from build123d import *

# Parameters (mm, degrees)
F1_DEPTH = 50.8
F2_R     = 7.58365402
F3_DEPTH = 38.1
F4_DEPTH = 38.1
F5_R     = 6.3202279554
F6_DEPTH = 76.2
F7_R     = 6.2629522454
F8_DEPTH = 50.8


with BuildPart() as f1:
    # F0 (on Top) → F1 (new body)
    with BuildSketch(Plane.XY):
        Polygon((-23.0499133468, 13.3078736756), (-23.0499133468, -13.3078736756), (0, -26.6157473511), (23.0499133468, -13.3078736756), (23.0499133468, 13.3078736756), (0, 26.6157473511), align=None)
        Polygon((0, -19.5391465708), (-16.9213972986, -9.7695732854), (-16.9213972986, 9.7695732854), (0, 19.5391465708), (16.9213972986, 9.7695732854), (16.9213972986, -9.7695732854), align=None, mode=Mode.SUBTRACT)
    extrude(amount=F1_DEPTH)

    # F2 (on Right) → F3 (cut)
    with BuildSketch(Plane.YZ):
        with Locations((0, 27.9511734843)):
            Circle(F2_R)
    extrude(amount=F3_DEPTH, mode=Mode.SUBTRACT)

    # F2 (on Right) → F4 (cut)
    with BuildSketch(Plane.YZ):
        with Locations((0, 27.9511734843)):
            Circle(F2_R)
    extrude(amount=-F4_DEPTH, mode=Mode.SUBTRACT)

    # F5 (on face) → F6 (cut)
    with BuildSketch(Plane(origin=(-11.5249566734, -19.9618105133, 0), x_dir=(0.8660254038, -0.5, 0), z_dir=(-0.5, -0.8660254038, 0))):
        with Locations((0, 24.6956739575)):
            Circle(F5_R)
    extrude(amount=-F6_DEPTH, mode=Mode.SUBTRACT)

    # F7 (on face) → F8 (cut)
    with BuildSketch(Plane(origin=(11.5249566734, -19.9618105133, 0), x_dir=(0.8660254038, 0.5, 0), z_dir=(0.5, -0.8660254038, 0))):
        with Locations((0, 26.1488687247)):
            Circle(F7_R)
    extrude(amount=-F8_DEPTH, mode=Mode.SUBTRACT)


solid = f1.part
Part model, mm, in its own coordinate system. A direction names the side the tool comes from. Coordinates: 2 decimals unless noted, no trailing zeros. Order: outer loops, then holes, each group sorted by start corner. A loop starts at its lowest first (then second) coordinate and runs counter-clockwise, first axis right, second up. Notation, with made-up numbers: M 8.25,20 L 14.25,20 A28 cw 14.25,56 Z; hole C 16,-36 d4. An arc over 180 degrees is marked long. One line per question, with ' | ' between items.
Q1. Slice it at B-B (y = -9). Give the cut face in (x, z), and give its area (3 significant figures).
A:
outline: M -23.05,0 L -16.92,0 L -16.92,50.8 L -23.05,50.8 Z; M 16.92,0 L 23.05,0 L 23.05,50.8 L 16.92,50.8 Z | area: 623 mm^2
Q2. Slice it at A-A (y = 0). Give the cut face in (x, z), and give its area (3 significant figures).
A:
outline: M -23.05,0 L -16.92,0 L -16.92,20.37 L -23.05,20.37 Z; M -23.05,35.53 L -16.92,35.53 L -16.92,50.8 L -23.05,50.8 Z; M 16.92,0 L 23.05,0 L 23.05,20.37 L 16.92,20.37 Z; M 16.92,35.53 L 23.05,35.53 L 23.05,50.8 L 16.92,50.8 Z | area: 437 mm^2
Q3. Drill centre lines: line 1 (X direction, y = 8.5, z = 4.5); line 2 (Z direction, x = -18, y = 0); line 3 (X direction, y = 11.5, z = 27). Where is each one in solid material? Low to high.
A:
line 1: x = -23.05 to -16.92, 16.92 to 23.05 | line 2: z = 0 to 20.37, 35.53 to 50.8 | line 3: x = -23.05 to -13.92, 13.92 to 23.05
Q4. Slice it at C-C (x = 1). Give the cut face in (y, z).
A:
outline: M -26.04,0 L -18.96,0 L -18.96,50.8 L -26.04,50.8 Z; M 18.96,0 L 26.04,0 L 26.04,50.8 L 18.96,50.8 Z
Q5. Pin check, flat tips, straight feed: P1, Ø4, axis at y = -18.5, z = 23, coming from the +X side; P2, Ø10, axis at x = 8, z = 10, coming from the -Y side; P3, Ø3, axis at y = -2, z = 23, coming from the -X side. Stop position of each tip, or through.
A:
P1: stops at x = 17.52 | P2: stops at y = -24.88 | P3: passes through
Q6. 3-axis set-ups, long thin cutter, end or side, ignore diameter. For faces 1 (the face through (2.7, 17.98, 25.04)), 2 (the face through (8.785, 17.956, 18.526)): which of +Z, -Z, +X, -X, +Y, -Y reach the whole face in a straight line?
A:
face 1: +Z, -Z | face 2: none
Q7. Two-plate mould, pull along Z, no slides. Class faces 3 (the face through (12.93, -15.66, 31.43)), 4 (the face through (-7, -16, 50.8)), 5 (the face through (23.05, 0, 19)): +Z half, -Z half, draft (parallel to the pull), parting line (faces both ways), or undercut.
A:
face 3: undercut | face 4: +Z half | face 5: draft
Q8. Slice it at D-D (z = 15). Give the cut face in (x, y).
A:
outline: M -23.05,-13.31 L 0,-26.62 L 23.05,-13.31 L 23.05,13.31 L 0,26.62 L -23.05,13.31 Z; hole M -16.92,-9.77 L 0,-19.54 L 16.92,-9.77 L 16.92,9.77 L 0,19.54 L -16.92,9.77 Z
